Check sheet for the drawn part. Datum: minimum x, y, z corner. Units: mm. Give positions to 0.01 mm unless a question says otherwise; leave off trailing zeros. Loops run counter-clockwise (first coordinate to the right, second up) from the corner with the lowest first, then second, coordinate; pieces in that order, holes last.
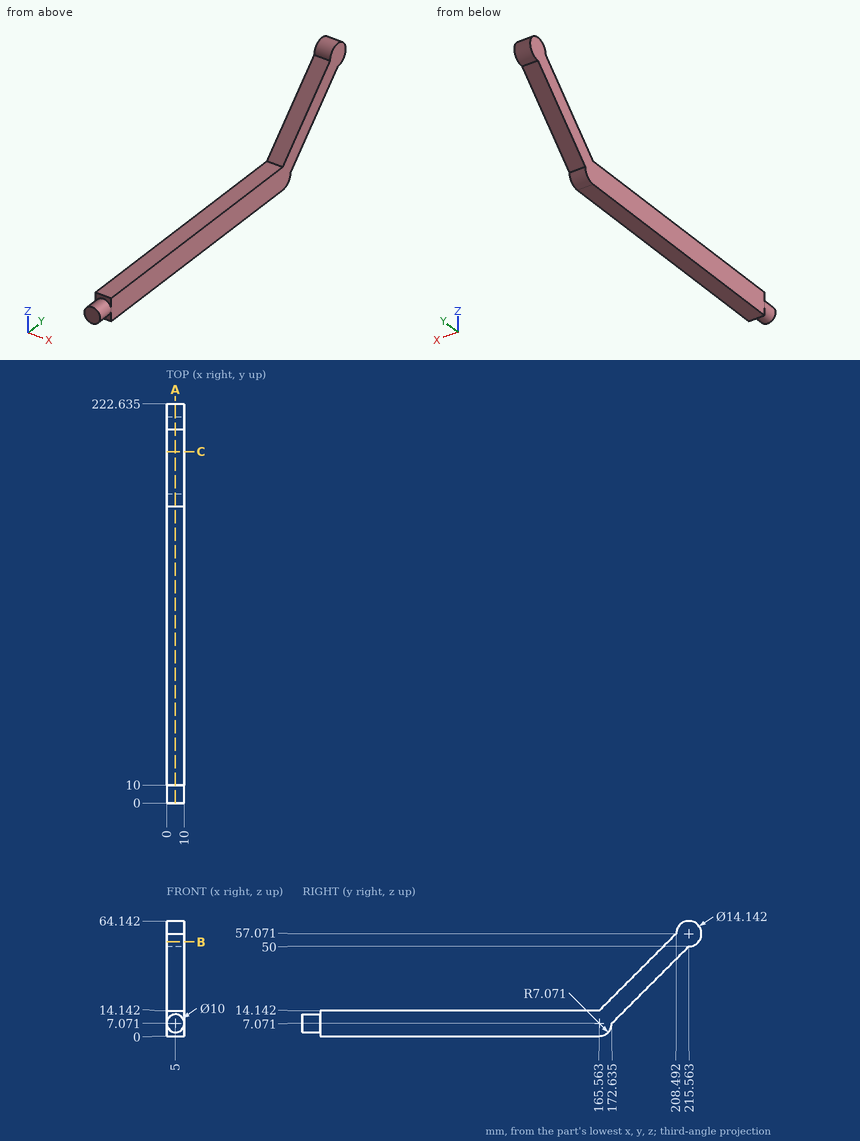
1) Sectioned sample at C-C on y = 196. Enter the section's corners in (x, z).
2) Sectioned sample at B-B on z = 52.5. Enter the section's corners in (x, y).
3) Scan lines: line 1 along Z through (x, y) = (4, 105); line 2 along Z through (x, y) = (7, 205.5) (1 decimal); line 3 along Y through (x, z) = (4, 55.5) (1 decimal). Record each from-to range of solid material in increasing order.
4) Depth check by flat-ended pin: P1, Ø1.5, axis at x = 3.5, z = 34.5, coming from the +Y side (1 decimal); P2, Ø1.5, axis at x = 8.5, z = 34.5, coming from the -Y side; P3, Ø1.5, axis at x = 9, z = 29, coming from the +Y side (1 decimal); P4, Ø5.5, axis at x = 4, z = 2, coming from the -Y side. Enter the tip coordinate at first touch or a pass-through.
5) Sectioned sample at A-A on x = 5. Enter the section's corners in (y, z) (1 decimal).
Determined:
1. outline: (0, 30.44) - (10, 30.44) - (10, 44.58) - (0, 44.58) - close
2. outline: (0, 203.92) - (10, 203.92) - (10, 220.96) - (0, 220.96) - close
3. line 1: z = 0 to 14.14
3. line 2: z = 39.9 to 54.1
3. line 3: y = 206.9 to 222.5
4. P1: stops at y = 200.8
4. P2: stops at y = 185.17
4. P3: stops at y = 195.3
4. P4: stops at y = 0
5. outline: (0, 2.1) - (10, 2.1) - (10, 0) - (165.6, 0) arc R7.1 ccw to (172.6, 7.1) - (215.6, 50) arc R7.1 ccw (long way) to (208.5, 57.1) - (165.6, 14.1) - (10, 14.1) - (10, 12.1) - (0, 12.1) - close
